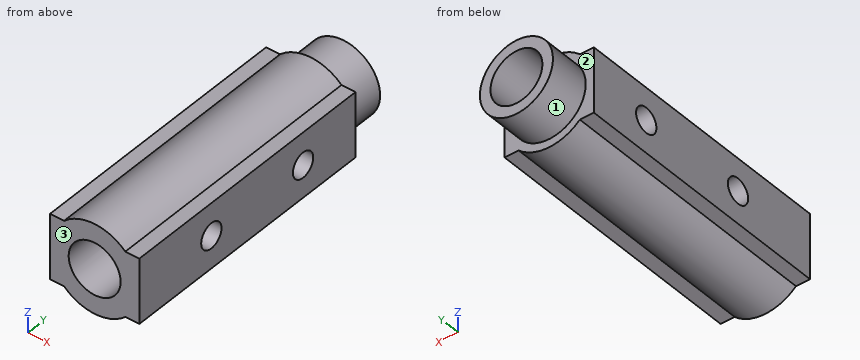
Autodesk Inventor part; units mm, degrees
ref_plane "YZ Plane" through (0, 0, 0) normal (1, 0, 0) x (0, 1, 0)
ref_plane "XZ Plane" through (0, 0, 0) normal (0, 1, 0) x (-1, 0, 0)
ref_plane "XY Plane" through (0, 0, 0) normal (0, 0, 1) x (1, 0, 0)
sketch "Sketch1" plane through (0, 0, 0) normal (0, 1, 0) x (-1, 0, 0)
  circle A0 centre (0, 0) radius 3.2
  circle A1 centre (0, 0) radius 5.5
  line L0 (0, 0) -> (0, -3.2)
  line L1 (0, 0) -> (0, 4)
  line L2 (-3.7749, 4) -> (-5.5, 4)
  line L3 (-5.5, 4) -> (-5.5, -4)
  line L4 (-5.5, -4) -> (-3.7749, -4)
  line L5 (0, -4) -> (0, 0)
  line L6 (3.7749, -4) -> (5.5, -4)
  line L7 (5.5, -4) -> (5.5, 4)
  line L8 (5.5, 4) -> (3.7749, 4)
  circle A2 centre (0, 0) radius 4.5
  dimension "d0" = 6.4
  dimension "d1" = 11
  dimension "d13" = 4
  dimension "d14" = 8
  dimension "d15" = 8
  dimension "d18" = 9
extrude "Extrusion3" add sketch "Sketch1" along normal blind 15 and the other way blind 18 contours A1 | L7 L6 A1 | A1 L8 L7 | A1 L3 L2 | L4 L3 A1 | A2
extrude "Extrusion4" add sketch "Sketch1" along normal blind 20 contours A2
sketch "Sketch3" plane through (5.5, -18, -4) normal (1, 0, 0) x (0, 0, -1)
  line L0 (0, 0) -> (0, 33)
  line L1 (0, 15) -> (-4, 15)
  line L2 (-4, 18) -> (-4, 11)
  line L3 (-4, 18) -> (-4, 25)
  circle A0 centre (-4, 25) radius 1.55
  circle A1 centre (-4, 11) radius 1.55
  dimension "d21" = 7
  dimension "d22" = 7
  dimension "d23" = 3.1
  dimension "d24" = 3.1
extrude "Extrusion5" cut sketch "Sketch3" against normal blind 20
properties part number "shaft_to_shaft_coupler"
Verification items for the finished model (mm, model axes). Face numbers are marked on the shaded views. Coordinates: 2 decimals unless noted, no trailing zeros. Write each loop counter-clockwise with the first axis right and the second up, starting at its lowest first coordinate (ties: lowest second). Pieces come first, ordered by that corner, then holes. Notation, with made-up numbers: (61.25, 19.5) -> (67.25, 19.5) arc R22 cw to (67.25, 50.5) -> close; hole circle Ø5 at (69.5, -27). An arc over 180 degrees is marked (long way). One line per item, written item: value. Start each with the question number.
Q1. Cross-section at C-C on y = -7. Enter the section's corners in (x, z), and give its area (3 significant figures).
Q2. Cross-section at B-B on x = 0. Enter the section's corners in (y, z), and give its area (3 significant figures).
Q3. Mould release check, pull along Y, two halves, no side actions. Record for the marked faces 1, 2 and 3: pulls with the +Y half, pulls with the -Y half, needs draft (parallel to the pull), parting line crosses it, or undercut.
Q4. Cross-section at A-A on z = 0. Enter the section's corners in (x, y), and give its area (3 significant figures).
Q5. Go/stop test with flat-tipped pins: P1, Ø1.9, axis at x = 5, y = -1, coming from the -Z side; P2, Ø0.9, axis at x = -5, y = -8.5, coming from the +Z side; P3, Ø4, axis at x = 2.5, y = -2.5, coming from the +Z side; P4, Ø4, axis at x = -1.5, y = 10.5, coming from the -Z side. Record where each tip stops, or that it passes through.
Q6. Cross-section at D-D on y = 12. Enter the section's corners in (x, z).
Q7. Thickness scan on L1, parallel to Y at x = -4.3, z = 0; L2, parallel to X at y = 12.5, z = 0; L3, parallel to Y at x = 4.7, z = 0. Record the ranges inside material, lowest first. Write a range as from..to.
Checked values:
1. outline: (-5.5, -4) -> (-3.77, -4) arc R5.5 ccw to (3.77, -4) -> (5.5, -4) -> (5.5, -1.55) -> (2.8, -1.55) arc R3.2 cw to (-2.8, -1.55) -> (-5.5, -1.55) -> close; (-5.5, 1.55) -> (-2.8, 1.55) arc R3.2 cw to (2.8, 1.55) -> (5.5, 1.55) -> (5.5, 4) -> (3.77, 4) arc R5.5 ccw to (-3.77, 4) -> (-5.5, 4) -> close
1. area: 56.3 mm²
2. outline: (-18, -5.5) -> (15, -5.5) -> (15, -4.5) -> (20, -4.5) -> (20, -3.2) -> (-18, -3.2) -> close; (-18, 3.2) -> (20, 3.2) -> (20, 4.5) -> (15, 4.5) -> (15, 5.5) -> (-18, 5.5) -> close
2. area: 165 mm²
3. face 1: needs draft
3. face 2: pulls with the +Y half
3. face 3: pulls with the -Y half
4. outline: (-5.5, -18) -> (-3.2, -18) -> (-3.2, -8.55) -> (-5.5, -8.55) -> close; (-5.5, -5.45) -> (-3.2, -5.45) -> (-3.2, 5.45) -> (-5.5, 5.45) -> close; (-5.5, 8.55) -> (-3.2, 8.55) -> (-3.2, 20) -> (-4.5, 20) -> (-4.5, 15) -> (-5.5, 15) -> close; (3.2, -18) -> (5.5, -18) -> (5.5, -8.55) -> (3.2, -8.55) -> close; (3.2, -5.45) -> (5.5, -5.45) -> (5.5, 5.45) -> (3.2, 5.45) -> close; (3.2, 8.55) -> (5.5, 8.55) -> (5.5, 15) -> (4.5, 15) -> (4.5, 20) -> (3.2, 20) -> close
4. area: 136 mm²
5. P1: stops at z = -4
5. P2: stops at z = 4
5. P3: stops at z = 5.48
5. P4: stops at z = -5.5
6. outline: (-5.5, -4) -> (-3.77, -4) arc R5.5 ccw to (3.77, -4) -> (5.5, -4) -> (5.5, 4) -> (3.77, 4) arc R5.5 ccw to (-3.77, 4) -> (-5.5, 4) -> close; hole circle Ø6.4 at (0, 0)
7. L1: y = -18..-8.55, -5.45..5.45, 8.55..20
7. L2: x = -5.5..-3.2, 3.2..5.5
7. L3: y = -18..-8.55, -5.45..5.45, 8.55..15
